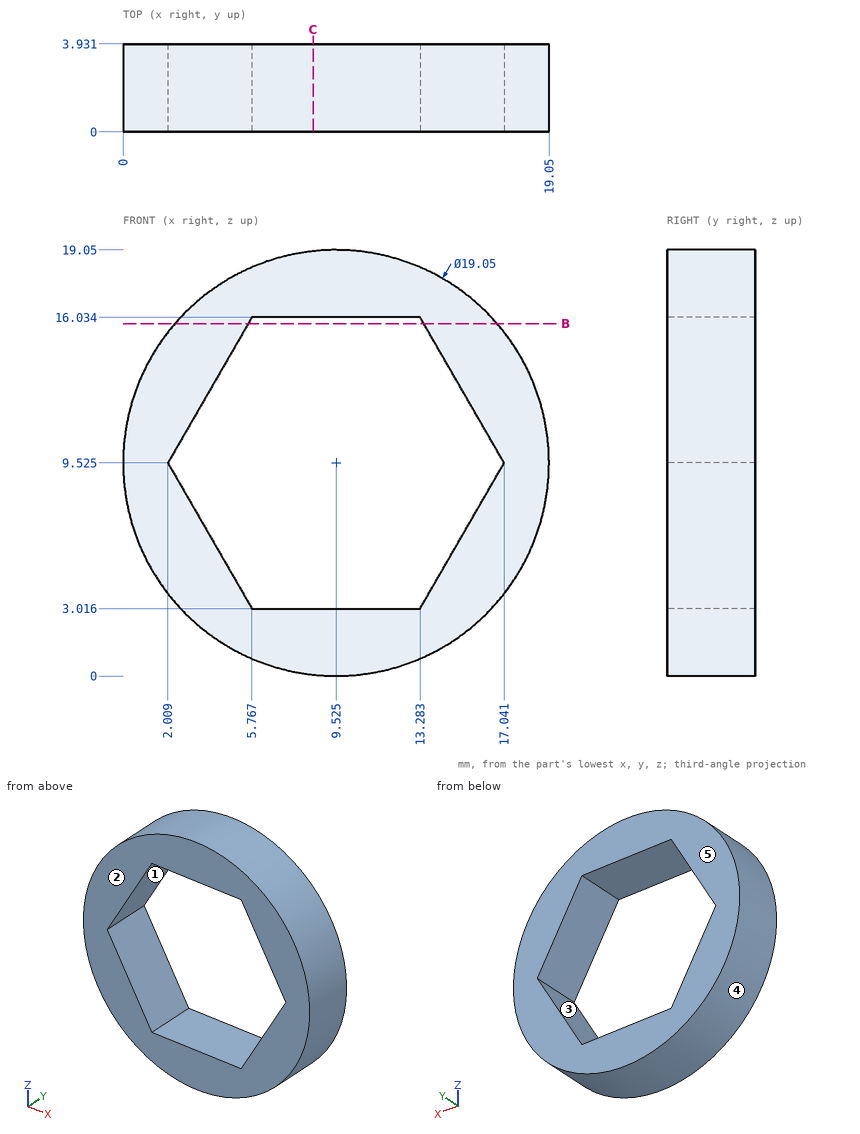
The drawing under review shows one solid part. Ordinate dimensions are in mm from its lowest x, y, z. A direction names the side the tool comes from. Round coordinates to 2 decimals unless told otherwise and drop trailing zeros. Write each loop counter-clockwise with the first axis right and the second up, starting at its lowest first coordinate (ties: lowest second). Pieces come first, ordered by that corner, then holes. Notation, with made-up numbers: (52, 15) -> (109, 15) arc R10 cw to (109, 27) -> close; hole circle Ø6 at (55.5, 50). An arc over 180 degrees is marked (long way). Put each result on its own line as item: value.
Q1. Clearance check with flat-ended pins moving along their axes: pin 1 Ø1 at (y, z) = (0.5, 6) entering from +X; pin 2 Ø3 at (x, z) = (6, 8) entering from +Y; pin 3 Ø1 at (x, y) = (3, 3) entering from +Z; pin 4 Ø2 at (x, y) = (11, 2.5) entering from +Z. State where each tip first meets the part, or that it passes through.
Determined:
pin 1: stops at x = 18.56
pin 2: passes through
pin 3: stops at z = 16.9
pin 4: stops at z = 19.04
Q2. The part is to be moulded in two halves that separate along X. For the marked faces 3, 4 and 5, say which applies: released by +X, released by -X, zero draft, split by the parting line, or undercut.
Determined:
face 3: undercut
face 4: split by the parting line
face 5: zero draft
Q3. Consider section C-C on x = 8.5. State the section outline as (y, z) points (1 decimal).
Determined:
outline: (0, 0.1) -> (3.9, 0.1) -> (3.9, 3) -> (0, 3) -> close; (0, 16) -> (3.9, 16) -> (3.9, 19) -> (0, 19) -> close
Q4. Machinability: for the marked faces 1 and 2, which of the approach directions +Z, -Z, +X, -X, +Y, -Y give a long, thin tool a straight path to every point of the face, cutting with its end or side? Answer none if there is none.
Determined:
face 1: +Y, -Y
face 2: +Z, -Z, +X, -X, -Y
Q5. Consider section B-B on z = 15.75. State the section outline as (x, y) points (1 decimal).
Determined:
outline: (2.3, 0) -> (5.6, 0) -> (5.6, 3.9) -> (2.3, 3.9) -> close; (13.4, 0) -> (16.7, 0) -> (16.7, 3.9) -> (13.4, 3.9) -> close
Q6. To check wall thickness, follow L1, parallel to Z at x = 5.25, y = 0.3 (1 decimal); L2, parallel to X at y = 3.55, z = 9.25 (1 decimal); L3, parallel to X at y = 0.35, z = 7.75 (1 decimal). State the ranges of each line that lie inside material, in increasing order. Write a range as [from, to].
Determined:
L1: z = [1, 3.9], [15.1, 18]
L2: x = [0, 2.2], [16.9, 19]
L3: x = [0.2, 3], [16, 18.9]
